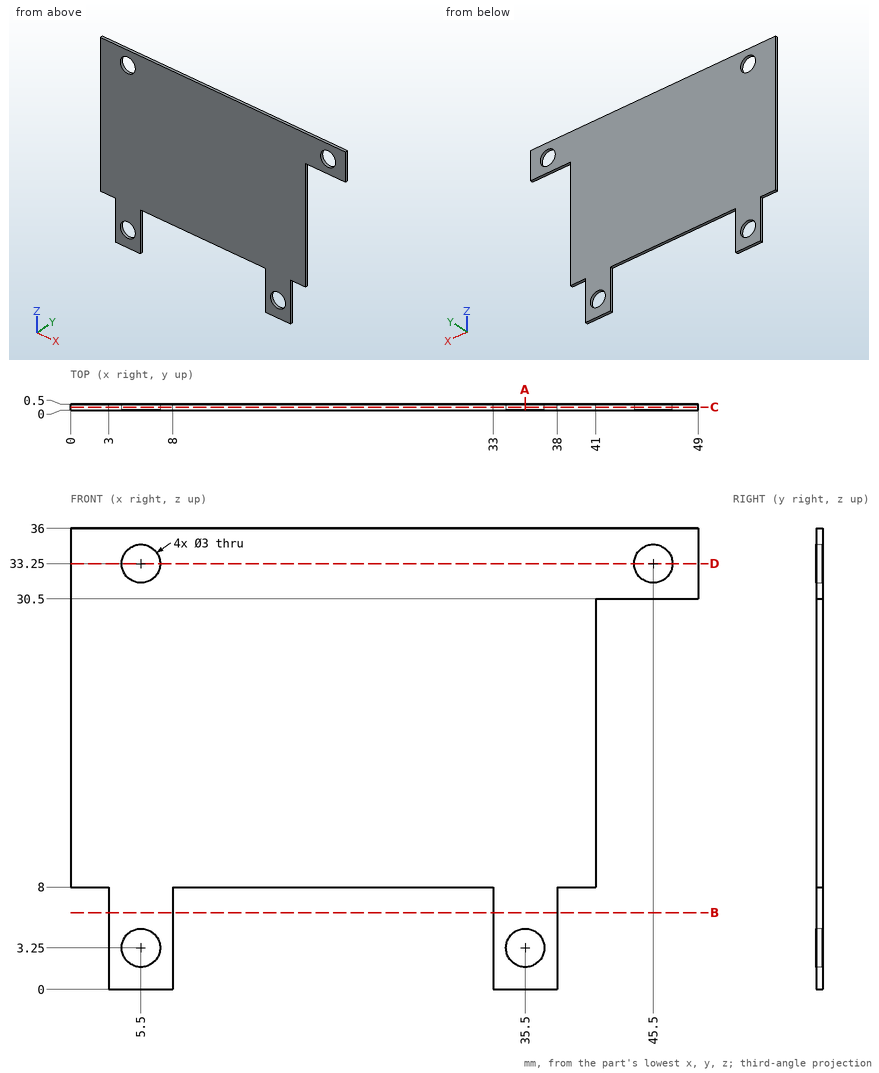
Job drawing, mm, ordinate dimensions from the low corner. One solid piece. Give positions to 0.01 mm unless a question says otherwise; leave off trailing zeros. Loops run counter-clockwise (first coordinate to the right, second up) from the corner with the lowest first, then second, coordinate; pieces in that order, holes last. Notation, with made-up numbers: M -29,-0.5 L 3,-0.5 A25 ccw 3,32.5 Z; hole C -23.5,41.25 d2. An arc over 180 degrees is marked long. Answer in a Markdown table with one row per item. Add a question column.
Item 1: Band-saw the part on C-C on y = 0.25. Give the cut face in (x, z), then the cut area to 3 significant figures.
Item 2: Probe probe 1 along X at (y, z) = (0.35, 33.25); probe 2 along Z at (x, y) = (5.5, 0.2); probe 3 along X at (y, z) = (0.2, 3.25). List the from-to ranges inside material, lowest first.
Item 3: Band-saw the part on D-D on z = 33.25. Give the cut face in (x, y).
Item 4: Band-saw the part on A-A on x = 35.5. Give the cut face in (y, z).
Item 5: Band-saw the part on B-B on z = 6. Give the cut face in (x, y).
Reply:
| question | item | result |
|---|---|---|
| 1 | outline | M 0,8 L 3,8 L 3,0 L 8,0 L 8,8 L 33,8 L 33,0 L 38,0 L 38,8 L 41,8 L 41,30.5 L 49,30.5 L 49,36 L 0,36 Z; hole C 5.5,3.25 d3; hole C 5.5,33.25 d3; hole C 35.5,3.25 d3; hole C 45.5,33.25 d3 |
| 1 | area | 1,240 mm^2 |
| 2 | probe 1 | x = 0 to 4, 7 to 44, 47 to 49 |
| 2 | probe 2 | z = 0 to 1.75, 4.75 to 31.75, 34.75 to 36 |
| 2 | probe 3 | x = 3 to 4, 7 to 8, 33 to 34, 37 to 38 |
| 3 | outline | M 0,0 L 4,0 L 4,0.5 L 0,0.5 Z; M 7,0 L 44,0 L 44,0.5 L 7,0.5 Z; M 47,0 L 49,0 L 49,0.5 L 47,0.5 Z |
| 4 | outline | M 0,0 L 0.5,0 L 0.5,1.75 L 0,1.75 Z; M 0,4.75 L 0.5,4.75 L 0.5,36 L 0,36 Z |
| 5 | outline | M 3,0 L 8,0 L 8,0.5 L 3,0.5 Z; M 33,0 L 38,0 L 38,0.5 L 33,0.5 Z |
